from build123d import *

# Parameters (mm, degrees)
SKETCH2_R                       = 30.5
CUT_EXTRUDE1_DEPTH              = 2
M3X0_5_TAPPED_HOLE1_D           = 2.5
M3X0_5_TAPPED_HOLE1_DEPTH       = 7.5
M3X0_5_TAPPED_HOLE1_TIP         = 0.751075774
M3X0_5_TAPPED_HOLE2_D           = 2.5
M3X0_5_TAPPED_HOLE2_DEPTH       = 7.5
M3X0_5_TAPPED_HOLE2_CSINK_D     = 3.05
M3X0_5_TAPPED_HOLE2_CSINK_ANGLE = 90
M3X0_5_TAPPED_HOLE2_TIP         = 0.751075774
M3X0_5_TAPPED_HOLE3_D           = 2.5
M3X0_5_TAPPED_HOLE3_DEPTH       = 7.5
M3X0_5_TAPPED_HOLE3_CSINK_D     = 3.05
M3X0_5_TAPPED_HOLE3_CSINK_ANGLE = 90
M3X0_5_TAPPED_HOLE3_TIP         = 0.751075774
SKETCH11_R                      = 6.5
CUT_EXTRUDE2_DEPTH              = 13.8


with BuildPart() as part:
    # Sketch1 → Revolve1 (revolve)
    with BuildSketch(Plane.XY, mode=Mode.PRIVATE) as revolve1_sk:
        Polygon((-7.9, 0), (7.9, 0), (7.9, 31.5), (-5.4, 31.5), (-7.9, 28), align=None)
    revolve(revolve1_sk.sketch.rotate(Axis((-7.9, 0, 0), (1, 0, 0)), 180), axis=Axis((-7.9, 0, 0), (1, 0, 0)))

    # Sketch2 → Cut-Extrude1 (cut)
    with BuildSketch(Plane(origin=(7.9, 0, 0), x_dir=(0, 0, -1), z_dir=(1, 0, 0))):
        with Locations(Location((0, 0, 0), (0, 0, 90))):
            Circle(SKETCH2_R)
    extrude(amount=-CUT_EXTRUDE1_DEPTH, mode=Mode.SUBTRACT)

    # M3x0.5 Tapped Hole1
    with Locations(Plane.ZY.offset(7.9)):
        with Locations((-15.556349186, 15.556349186), (15.556349186, 15.556349186), (15.556349186, -15.556349186), (-15.556349186, -15.556349186)):
            Hole(M3X0_5_TAPPED_HOLE1_D / 2, depth=M3X0_5_TAPPED_HOLE1_DEPTH)
            with Locations((0, 0, -(M3X0_5_TAPPED_HOLE1_DEPTH + M3X0_5_TAPPED_HOLE1_TIP / 2))):  # 118° drill point
                Cone(0, M3X0_5_TAPPED_HOLE1_D / 2, M3X0_5_TAPPED_HOLE1_TIP, mode=Mode.SUBTRACT)

    # M3x0.5 Tapped Hole2
    with Locations(Plane.ZY.offset(7.9)):
        with Locations((-10.606601718, 10.606601718), (-10.606601718, -10.606601718), (10.606601718, -10.606601718), (10.606601718, 10.606601718)):
            CounterSinkHole(M3X0_5_TAPPED_HOLE2_D / 2, M3X0_5_TAPPED_HOLE2_CSINK_D / 2, depth=M3X0_5_TAPPED_HOLE2_DEPTH, counter_sink_angle=M3X0_5_TAPPED_HOLE2_CSINK_ANGLE)
            with Locations((0, 0, -(M3X0_5_TAPPED_HOLE2_DEPTH + M3X0_5_TAPPED_HOLE2_TIP / 2))):  # 118° drill point
                Cone(0, M3X0_5_TAPPED_HOLE2_D / 2, M3X0_5_TAPPED_HOLE2_TIP, mode=Mode.SUBTRACT)

    # M3x0.5 Tapped Hole3
    with Locations(Plane.ZY.offset(7.9)):
        with Locations((0, 12.5), (-12.5, 0), (0, -12.5), (12.5, 0)):
            CounterSinkHole(M3X0_5_TAPPED_HOLE3_D / 2, M3X0_5_TAPPED_HOLE3_CSINK_D / 2, depth=M3X0_5_TAPPED_HOLE3_DEPTH, counter_sink_angle=M3X0_5_TAPPED_HOLE3_CSINK_ANGLE)
            with Locations((0, 0, -(M3X0_5_TAPPED_HOLE3_DEPTH + M3X0_5_TAPPED_HOLE3_TIP / 2))):  # 118° drill point
                Cone(0, M3X0_5_TAPPED_HOLE3_D / 2, M3X0_5_TAPPED_HOLE3_TIP, mode=Mode.SUBTRACT)

    # Sketch11 → Cut-Extrude2 (cut)
    with BuildSketch(Plane.ZY.offset(7.9)):
        with Locations(Location((0, 0, 0), (0, 0, 270))):
            Circle(SKETCH11_R)
    extrude(amount=-CUT_EXTRUDE2_DEPTH, mode=Mode.SUBTRACT)


solid = part.part
Model file for the job. Use its own axes, mm. A direction names the side the tool comes from. Give positions to 0.01 mm unless a question says otherwise; leave off trailing zeros. Order: outer loops, then holes, each group sorted by start corner. A loop starts at its lowest first (then second) coordinate and runs counter-clockwise, first axis right, second up. Notation, with made-up numbers: (67.5, 14.25) - (98.5, 14.25) arc R25 cw to (98.5, 46.25) - close; hole circle Ø6 at (80.25, 12). An arc over 180 degrees is marked (long way). Write item = value, one per line. Start each with the question number.
1. Drop flat-ended pins along their axis: P1, Ø8, axis at x = -4.5, z = -18.5, coming from the +Y side; P2, Ø2, axis at y = 10.61, z = 10.61, coming from the +X side; P3, Ø4, axis at x = 4, y = -12, coming from the +Z side; P4, Ø3, axis at x = -1.5, z = -1, coming from the +Y side. Give the stop position or say it passes through.
2. Which spindle directions (+Z, -Z, +X, -X, +Y, -Y) get a long thin tool onto all of the face, cutting with end or side? Do faces 1 (the cylindrical face through (-1.097, 5.158, -3.955)), 2 (the cylindrical face through (-3.96, 0.05, -11.25)), 3 (the flat face through (5.9, 0, 7)). Say none if no direction does.
3. Probe line 1 along Z through (x, y) = (-1.75, 0); line 2 along Z through (x, y) = (7.25, 0); line 3 along Y through (x, z) = (-5.25, 9.5). List the from-to ranges inside material, lowest first.
4. Cut at A-A, the plane x = -1.5. State how many separate pieces and enclosed holes the cut face has, and give its area (3 significant figures).
5. Cut at B-B, the plane x = 6.75. List the corners of the cut face in (y, z), and give its area (3 significant figures).
6. Two-plate mould, pull along Y, no slides. Class faces 4 (the cylindrical face through (-3.962, -11.827, 10.878)), 5 (the conical face through (-7.78, -26.87, -8.46)): pulls with the +Y half, pulls with the -Y half, needs draft (parallel to the pull), parting line crosses it, or undercut.
Taken from the geometry:
q1.P1 = 27.96
q1.P2 = 5.9
q1.P3 = 29.87
q1.P4 = 31.5
q2.face_1 = +X, -X
q2.face_2 = -X
q2.face_3 = +X
q3.line_1 = -31.5 to -13.75, -11.25 to -6.5, 6.5 to 11.25, 13.75 to 31.5
q3.line_2 = -31.5 to -30.5, 30.5 to 31.5
q3.line_3 = -30.03 to -11.19, -10.03 to 10.03, 11.19 to 30.03
q4.separate_pieces = 1
q4.enclosed_holes = 13
q4.area = 2,930 mm²
q5.outline = circle Ø63 at (0, 0); hole circle Ø61 at (0, 0)
q5.area = 195 mm²
q6.face_4 = undercut
q6.face_5 = parting line crosses it
